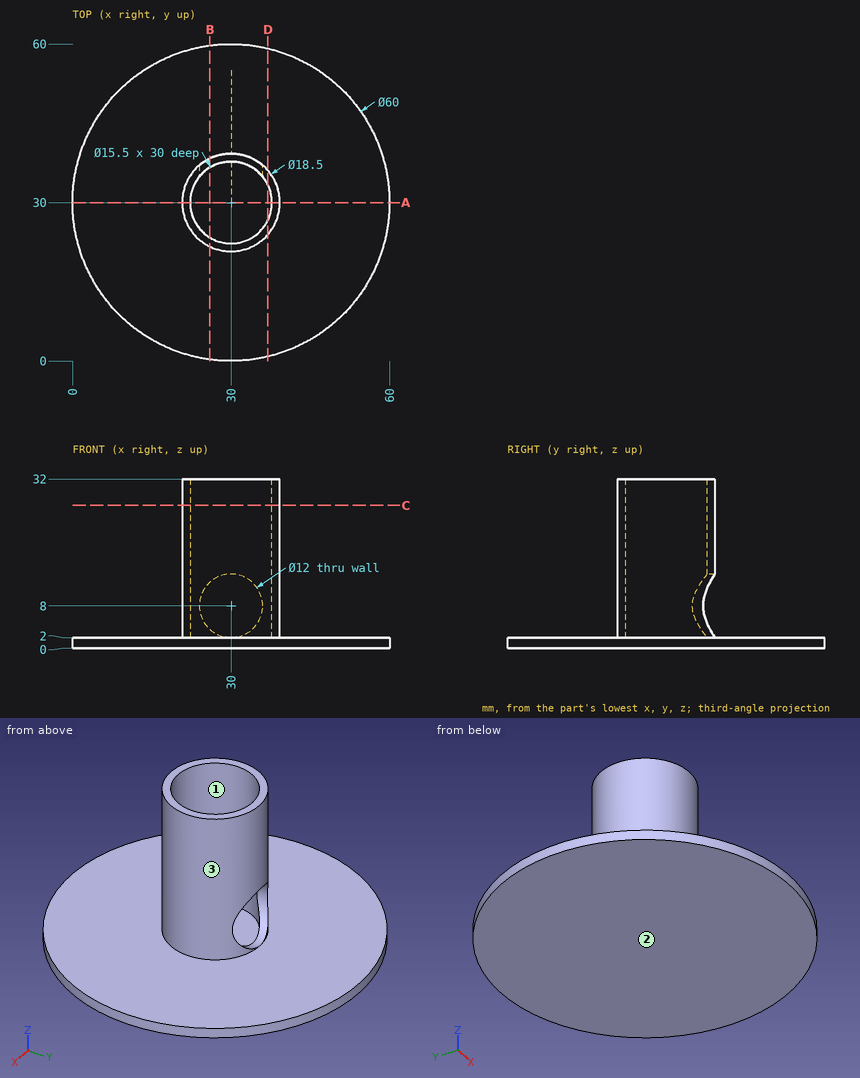
Check sheet for the drawn part. Datum: minimum x, y, z corner. Units: mm. Give positions to 0.01 mm unless a question says otherwise; leave off trailing zeros. Order: outer loops, then holes, each group sorted by start corner. A loop starts at its lowest first (then second) coordinate and runs counter-clockwise, first axis right, second up. Notation, with made-up numbers: (25.25, -5.5) - (73.25, -5.5) arc R12 ccw to (73.25, 16.5) - close; hole circle Ø11 at (63.5, -40). An arc over 180 degrees is marked (long way). Answer as a JSON object with one key per item and string values.
(1) Cross-section at D-D (x = 37). Record the cut outline in (y, z), then the cut area to 3 significant figures.
Report:
{"outline": "(0.83, 0) - (59.17, 0) - (59.17, 2) - (36.05, 2) - (36.05, 32) - (33.33, 32) - (33.33, 2) - (26.67, 2) - (26.67, 32) - (23.95, 32) - (23.95, 2) - (0.83, 2) - close", "area": "280 mm^2"}
(2) Cross-section at B-B (x = 26). Record the cut outline in (y, z).
Report:
{"outline": "(0.27, 0) - (59.73, 0) - (59.73, 2) - (38.34, 2) - (38.34, 3.53) - (36.64, 3.53) - (36.64, 2) - (23.36, 2) - (23.36, 32) - (21.66, 32) - (21.66, 2) - (0.27, 2) - close; (36.64, 12.47) - (38.34, 12.47) - (38.34, 32) - (36.64, 32) - close"}
(3) Cross-section at A-A (y = 30). Record the cut outline in (x, z).
Report:
{"outline": "(0, 0) - (60, 0) - (60, 2) - (39.25, 2) - (39.25, 32) - (37.75, 32) - (37.75, 2) - (22.25, 2) - (22.25, 32) - (20.75, 32) - (20.75, 2) - (0, 2) - close"}
(4) Material ranges on line 1 (Z direction, x = 23, y = 19); line 2 (X direction, y = 30, z = 20); line 3 (Y direction, x = 36, z = 5), recorded low to high.
Report:
{"line 1": "0 to 2", "line 2": "20.75 to 22.25, 37.75 to 39.25", "line 3": "22.96 to 25.09, 34.91 to 37.04"}
(5) Cross-section at C-C (z = 27). Record the cut outline in (x, y).
Report:
{"outline": "circle Ø18.5 at (30, 30); hole circle Ø15.5 at (30, 30)"}
(6) Depth check by flat-ended pin: pin 1 Ø14 at (x, y) = (30, 30) entering from +Z; pin 2 Ø8 at (y, z) = (22, 18) entering from +X; pin 3 Ø7 at (x, z) = (30, 8) entering from +Y; pin 4 Ø6 at (x, z) = (15, 24) entering from -Y. Enter the tip coordinate at first touch or a pass-through.
Report:
{"pin 1": "z = 2", "pin 2": "x = 38.34", "pin 3": "y = 23.09", "pin 4": "through"}
(7) Draft check along Y on the marked faces 1, 2 and 3. Enter one of: released by +Y, released by -Y, zero draft, split by the parting line, or undercut.
Report:
{"face 1": "undercut", "face 2": "zero draft", "face 3": "split by the parting line"}
